Answer from the drawing. Dimensions are ordinates in mm from the lowest x, y and z of the part. Coordinates: 2 decimals unless noted, no trailing zeros. Write each loop counter-clockwise with the first axis right and the second up, starting at its lowest first coordinate (ties: lowest second). Pieces come first, ordered by that corner, then holes.
(1) The part is cut by section B-B on x = 5. Determine the outline of the cut face in (y, z), plus the area to 3 significant figures.
(2) The part is cut by section D-D on z = 23. Determine the outline of the cut face in (x, y), plus the area to 3 significant figures.
(3) Straight lines are drawn through the part: line 1 (X direction, y = 1.45, z = 11); line 2 (Z direction, x = 4, y = 3.2); line 3 (Z direction, x = 19.75, y = 0.75). For each, find the intervals that lie inside material, in ascending order.
(4) The part is cut by section C-C on y = 2.55. Determine the outline of the cut face in (x, z).
(5) For a pull along X with two mould halves and no side action, classify the marked faces 1, 2 and 3 as +X half, -X half, draft (parallel to the pull), parting line (faces both ways), or undercut.
(6) The part is cut by section A-A on z = 31. Determine the outline of the cut face in (x, y), plus the area to 3 significant figures.
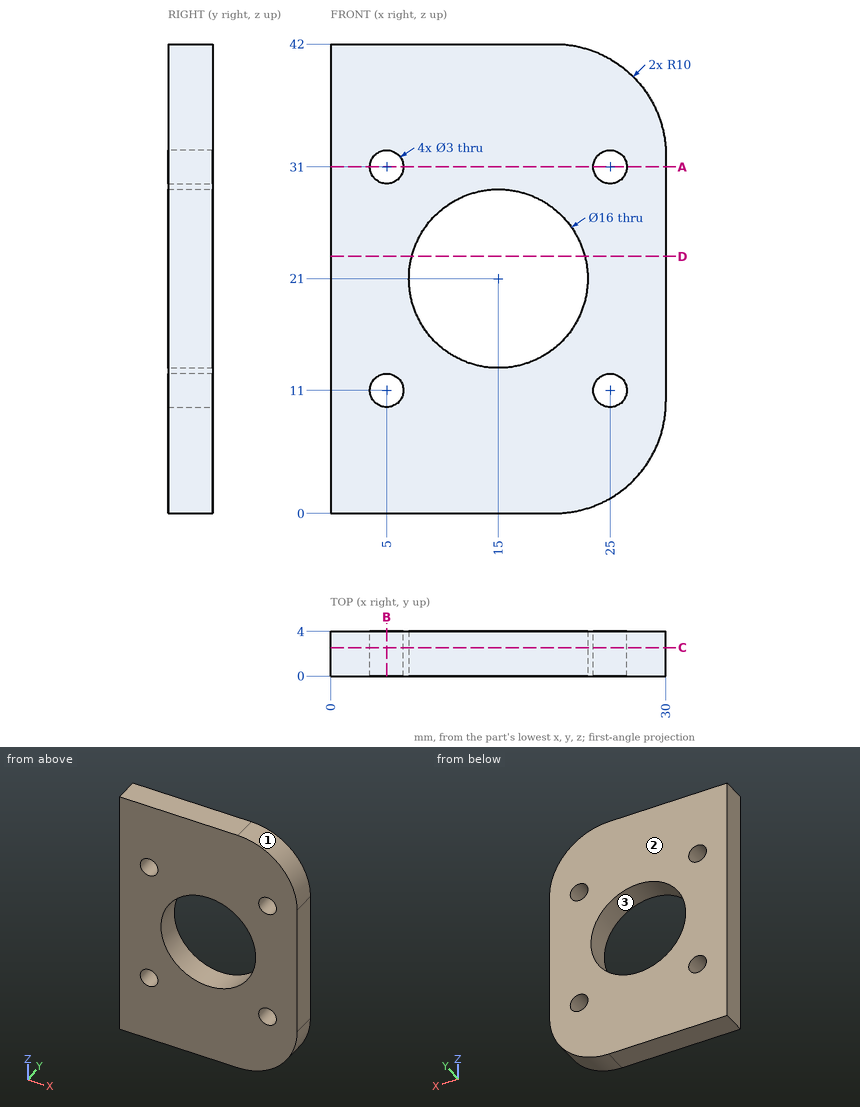
Model answer:
1. outline: (0, 0) - (4, 0) - (4, 9.5) - (0, 9.5) - close; (0, 12.5) - (4, 12.5) - (4, 29.5) - (0, 29.5) - close; (0, 32.5) - (4, 32.5) - (4, 42) - (0, 42) - close
1. area: 144 mm2
2. outline: (0, 0) - (7.25, 0) - (7.25, 4) - (0, 4) - close; (22.75, 0) - (30, 0) - (30, 4) - (22.75, 4) - close
2. area: 58.0 mm2
3. line 1: x = 0 to 3.5, 6.5 to 23.5, 26.5 to 30
3. line 2: z = 0 to 9.88, 12.12 to 29.88, 32.12 to 42
3. line 3: z = 0 to 14.56, 27.44 to 42
4. outline: (0, 0) - (20, 0) arc R10 ccw to (30, 10) - (30, 32) arc R10 ccw to (20, 42) - (0, 42) - close; hole circle Ø3 at (5, 11); hole circle Ø3 at (5, 31); hole circle Ø16 at (15, 21); hole circle Ø3 at (25, 11); hole circle Ø3 at (25, 31)
5. face 1: +X half
5. face 2: draft
5. face 3: undercut
6. outline: (0, 0) - (3.5, 0) - (3.5, 4) - (0, 4) - close; (6.5, 0) - (23.5, 0) - (23.5, 4) - (6.5, 4) - close; (26.5, 0) - (30, 0) - (30, 4) - (26.5, 4) - close
6. area: 96.0 mm2
